Check sheet for the drawn part. Datum: minimum x, y, z corner. Units: mm. A direction names the side the tool comes from. Round coordinates to 2 decimals unless told otherwise and drop trailing zeros. Write each loop counter-clockwise with the first axis right and the second up, starting at its lowest first coordinate (ties: lowest second). Pieces come first, ordered by that corner, then holes.
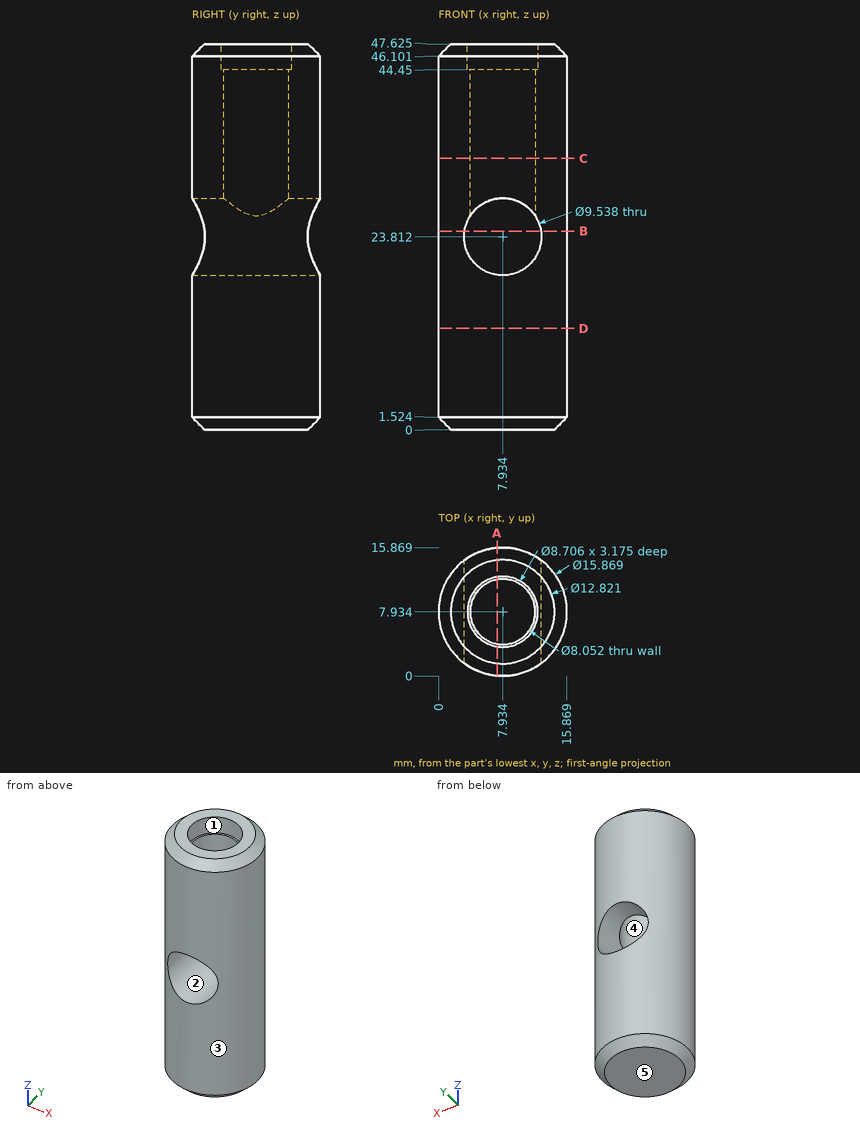
Q1. Release check for a two-part mould opening along Y. For the marked faces 3, 4 and 5 record: released by +Y, released by -Y, zero draft, split by the parting line, or undercut.
Recorded:
face 3: split by the parting line
face 4: undercut
face 5: zero draft
Q2. Tool access check on the marked faces 1 and 2. Record the directions out of +Z, -Z, +X, -X, +Y, -Y that give a thin tool (end or side, any length) a straight path to the whole face; none if there is none.
Recorded:
face 1: +Z
face 2: +Y, -Y
Q3. Sectioned sample at A-A (x = 7.25). Give the number of separate pieces and of enclosed holes in the cut face.
Recorded:
separate pieces: 3
enclosed holes: 0
Q4. Material ranges on line 1 along Z through (x, y) = (5.5, 3.75) (1 decimal); line 2 along Z through (x, y) = (8.25, 9) (1 decimal); line 3 along Y through (x, z) = (6.25, 45), recorded low to high.
Recorded:
line 1: z = 0 to 19.7, 27.9 to 47.6
line 2: z = 0 to 19.1
line 3: y = 0.18 to 3.92, 11.95 to 15.69
Q5. Sectioned sample at C-C (z = 33.5). Enter the section's corners in (x, y) (1 decimal).
Recorded:
outline: circle Ø15.9 at (7.9, 7.9); hole circle Ø8.1 at (7.9, 7.9)
Q6. Sectioned sample at B-B (z = 24.5). Enter the section's corners in (x, y) (1 decimal).
Recorded:
outline: (3.2, 1.6) - (3.2, 14.3) arc R7.9 ccw to start; (12.7, 1.6) arc R7.9 ccw to (12.7, 14.3) - close
Q7. Depth check by flat-ended pin: P1, Ø8, axis at x = 4.5, z = 11.5, coming from the -Y side; P2, Ø1, axis at x = 4.5, z = 19.5, coming from the -Y side; P3, Ø2.5, axis at x = 8.5, y = 8, coming from the +Z side; P4, Ø5, axis at x = 7.93, y = 7.93, coming from the +Z side (1 decimal). Enter the tip coordinate at first touch or a pass-through.
Recorded:
P1: stops at y = 0
P2: stops at y = 0.56
P3: stops at z = 19.4
P4: stops at z = 19.8
Q8. Sectioned sample at D-D (z = 12.5). Enter the section's corners in (x, y) (1 decimal).
Recorded:
outline: circle Ø15.9 at (7.9, 7.9)
